Autodesk Inventor part; units mm, degrees
ref_plane "YZ Plane" through (0, 0, 0) normal (1, 0, 0) x (0, 1, 0)
ref_plane "XZ Plane" through (0, 0, 0) normal (0, 1, 0) x (-1, 0, 0)
ref_plane "XY Plane" through (0, 0, 0) normal (0, 0, 1) x (1, 0, 0)
sketch "Sketch1" plane through (0, 0, 0) normal (0, 1, 0) x (-1, 0, 0)
  line L0 (0, 0) -> (12.7, 0)
  line L1 (12.7, 0) -> (12.7, -25.4)
  line L2 (12.7, -25.4) -> (0, -25.4)
  line L3 (0, -25.4) -> (0, 0)
  dimension "d1" = 25.4
  dimension "d2" = 12.7
extrude "Extrusion1" add sketch "Sketch1" along normal blind 45
sketch "Sketch7" plane through (0, 45, 0) normal (0, 1, 0) x (1, 0, 0)
  line L0 (-12.7, 0) -> (0, 0)
  line L1 (-12.7, 25.4) -> (-12.7, 0)
  line L2 (0, 0) -> (-12.7, 0)
  line L3 (-12.7, 0) -> (-12.7, 25.4)
  line L4 (-12.7, 25.4) -> (0, 25.4)
  line L5 (0, 25.4) -> (0, 0)
extrude "Extrusion6" add sketch "Sketch7" along normal blind 15
sketch "Sketch12" plane through (0, 60, 0) normal (0, 1, 0) x (1, 0, 0)
  line L0 (0, 0) -> (0, 25.4)
  line L1 (-12.7, 25.4) -> (-12.7, 0)
  line L2 (0, 4.8) -> (-12.7, 4.8)
  line L3 (-12.7, 4.8) -> (-12.7, 25.4)
  line L4 (-12.7, 25.4) -> (0, 25.4)
  line L5 (0, 25.4) -> (0, 4.8)
  point P0 (-12.7, 4.8)
  point P1 (-12.7, 4.8)
extrude "Extrusion11" cut sketch "Sketch12" against normal blind 9.216
fillet "Fillet5" radius 10.3 1 edges at (-6.35, 50.784, -25.4)
sketch "Sketch14" plane through (-12.7, 0, 0) normal (0, 0, 1) x (1, 0, 0)
  line L0 (0, 60) -> (12.7, 60)
  line L1 (12.7, 0) -> (12.7, 40.484)
  line L2 (0, 60) -> (12.7, 60)
  line L3 (12.7, 60) -> (12.7, 0)
  line L4 (12.7, 0) -> (0, 0)
  line L5 (0, 0) -> (0, 60)
extrude "Extrusion13" cut sketch "Sketch14" against normal blind 4.8
fillet "Fillet6" radius 10.3 1 edges at (-6.35, 50.784, -4.8)
sketch "Sketch18" plane through (0, 0, -25.4) normal (1, 0, 0) x (0, 0, -1)
  arc A0 (0, 40.484) -> (-20.6, 40.484) centre (-10.3, 40.484) ccw
  circle A1 centre (-10.3, 40.484) radius 3.175
  point P0 (-25.4, 0)
  dimension "d65" = 6.35
extrude "Extrusion17" cut sketch "Sketch18" against normal through all
properties part number "gear support"
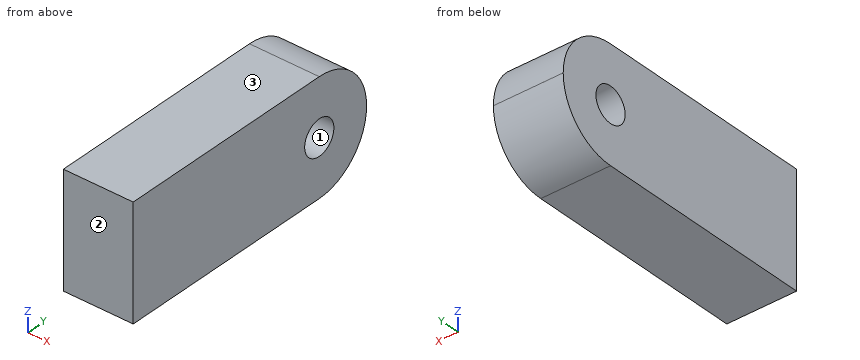
Check sheet for the modelled part. Datum: model origin and axes. Units: mm. Face numbers are marked on the shaded views. Round coordinates to 2 decimals unless told otherwise and drop trailing zeros. Order: outer loops, then holes, each group sorted by start corner. A loop starts at its lowest first (then second) coordinate and runs counter-clockwise, first axis right, second up.
1) Go/stop test with flat-tipped pins: pin 1 Ø1 at (y, z) = (24, -19.5) entering from +X; pin 2 Ø4 at (y, z) = (40.484, -15.1) entering from -X (1 decimal); pin 3 Ø6 at (x, z) = (-9, -19) entering from +Y. Record where each tip stops, or that it passes through.
2) Section check B-B (z = -12.5). Record the boundary of the cut face in (x, y).
3) Section check C-C (z = -10). Record the boundary of the cut face in (x, y).
4) Section check D-D (z = -23.5). Record the boundary of the cut face in (x, y).
5) Mould release check, pull along Z, two halves, no side actions. Record for the marked faces 1, 2 and 3: +Z half, -Z half, draft (parallel to the pull), parting line (faces both ways), or undercut.
6) Scan lines: line 1 (Y direction, x = -7, z = -15.1); line 2 (Z direction, x = -3.25, y = 40); line 3 (Z direction, x = -3, y = 39). Record each from-to range of solid material in increasing order.
Result:
1. pin 1: stops at x = 0
1. pin 2: passes through
1. pin 3: stops at y = 50.74
2. outline: (-12.7, 0) - (0, 0) - (0, 38.66) - (-12.7, 38.66) - close; (-12.7, 42.31) - (0, 42.31) - (0, 50.45) - (-12.7, 50.45) - close
3. outline: (-12.7, 0) - (0, 0) - (0, 49.43) - (-12.7, 49.43) - close
4. outline: (-12.7, 0) - (0, 0) - (0, 46.44) - (-12.7, 46.44) - close
5. face 1: undercut
5. face 2: draft
5. face 3: +Z half
6. line 1: y = 0 to 37.31, 43.66 to 50.78
6. line 2: z = -25.4 to -18.24, -11.96 to -4.8
6. line 3: z = -25.4 to -17.91, -12.29 to -4.8
